Geometry: final body of the model. Coordinates: model frame, mm. Give positions to 0.01 mm unless a question says otherwise; leave off trailing zeros. Order: outer loops, then holes, each group sorted by start corner. A loop starts at its lowest first (then second) coordinate and runs counter-clockwise, first axis right, second up. Notation, with made-up numbers: (49, -8.5) - (82, -8.5) arc R29 ccw to (82, 18.5) - close; hole circle Ø5 at (47, -26). An arc over 180 degrees is marked (long way). Use one line per item in the form item = value.
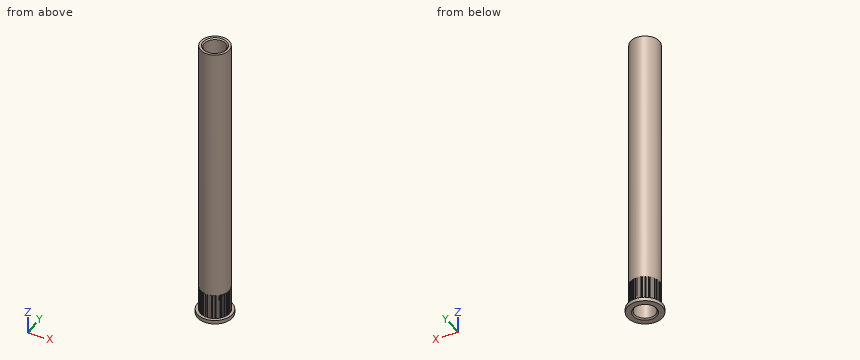
from build123d import *

# Parameters (mm, degrees)
F2_R            = 0.25
F3_DEPTH        = 20
F3_COPIES_COUNT = 60
F4_SIZE         = 1


# Not quite as in the source:
# - a pattern or mirror of a feature is missing from the dataset's text; its kind, count and spacing are read off the source's solid


with BuildPart() as f1:
    # F0 (on Front) → F1 (revolve)
    with BuildSketch(Plane.XZ):
        Polygon((-14, 0), (-8.5, 0), (-8.5, 233), (-11.5, 233), (-11.5, 3), (-14, 3), align=None)
    revolve(axis=Axis((0, 0, 48.0585359184), (0, 0, 1)))

    # F2 (on face) → F3 (join)
    with BuildSketch(Plane.XY.offset(3)):
        with Locations((0, -11.5)):
            Circle(F2_R)
    f3 = extrude(amount=F3_DEPTH)

    # F3_copies: F3 ×60 about axis
    f3_copies_axis = Axis((0, 0, 0), (0, 0, 1))
    for i in range(1, F3_COPIES_COUNT):
        add(f3.rotate(f3_copies_axis, i * 360 / F3_COPIES_COUNT))

    # F4
    f4_edges = [f1.edges().sort_by_distance(p)[0] for p in [
        (8.5, 0, 0),
        (8.5, 0, 233),
    ]]
    chamfer(f4_edges, length=F4_SIZE)


solid = f1.part
(1) Cut plane A-A on z = 139.5. Output: boundary loops of the cut face in (x, y), plus the area to 3 significant figures.
Computed values:
outline = circle Ø23 at (0, 0); hole circle Ø17 at (0, 0)
area = 188 mm²
(2) Contact query for flat-ended pins moving along their axis: pin 1 Ø4 at (x, z) = (-9, 127.5) entering from -Y; pin 2 Ø8 at (x, y) = (10.5, -8) entering from -Z; pin 3 Ø6 at (x, z) = (0, 56.5) entering from -Y; pin 4 Ø8 at (y, z) = (5.5, 85.5) entering from -X. Output: stop coordinate, or through.
Computed values:
pin_1 = -9.12
pin_2 = 0
pin_3 = -11.5
pin_4 = -11.4
(3) Ray query, line 1 along X through (y, z) = (0, 127); line 2 along Y through (x, z) = (6, 35). Return the intervals inside material, ascending.
Computed values:
line_1 = -11.5 to -8.5, 8.5 to 11.5
line_2 = -9.81 to -6.02, 6.02 to 9.81
